Input: part model. Units: mm. Frame: model coordinates. Face numbers are marked on the shaded views. Round coordinates to 2 decimals unless told otherwise and drop trailing zeros. Answer as CSV lines item,"result". Start each with the question number.
1) Line query: L1, parallel to Z at x = -240, y = 2.7. Output: solid intervals per line, ascending.
2) Mould query, pull axis Y, two halves, no side actions, for the marked faces 1 and 2. Classes: +Y half, -Y half, draft (parallel to the pull), parting line (faces both ways), or undercut.
3) First-contact query: P1, Ø6.5, axis at x = 160, z = -100, coming from the -Y side; P2, Ø9, axis at x = 320, z = -100, coming from the -Y side. Flat tips, straight axial feed; report the tip coordinate or a pass-through.
```python
from build123d import *

# Parameters (mm, degrees)
SKETCH1_W                                    = 760
SKETCH1_H                                    = 250
BOSS_EXTRUDE1_DEPTH                          = 3
CSK_FOR_M5_COUNTERSUNK_FLAT_HEAD_SCR_2_COUNT = 2
CSK_FOR_M5_COUNTERSUNK_FLAT_HEAD_SCR_2_PITCH = 80
CSK_FOR_M5_COUNTERSUNK_FLAT_HEAD_SCR_3_COUNT = 2
CSK_FOR_M5_COUNTERSUNK_FLAT_HEAD_SCR_3_PITCH = 160
CSK_FOR_M5_COUNTERSUNK_FLAT_HEAD_SCR_4_COUNT = 2
CSK_FOR_M5_COUNTERSUNK_FLAT_HEAD_SCR_4_PITCH = 240
CSK_FOR_M5_COUNTERSUNK_FLAT_HEAD_SCR_5_COUNT = 2
CSK_FOR_M5_COUNTERSUNK_FLAT_HEAD_SCR_5_PITCH = 320
CSK_FOR_M5_COUNTERSUNK_FLAT_HEAD_SCR_6_COUNT = 2
CSK_FOR_M5_COUNTERSUNK_FLAT_HEAD_SCR_6_PITCH = 80
CSK_FOR_M5_COUNTERSUNK_FLAT_HEAD_SCR_7_COUNT = 2
CSK_FOR_M5_COUNTERSUNK_FLAT_HEAD_SCR_7_PITCH = 160
CSK_FOR_M5_COUNTERSUNK_FLAT_HEAD_SCR_8_COUNT = 2
CSK_FOR_M5_COUNTERSUNK_FLAT_HEAD_SCR_8_PITCH = 240
CSK_FOR_M5_COUNTERSUNK_FLAT_HEAD_SCR_9_COUNT = 2
CSK_FOR_M5_COUNTERSUNK_FLAT_HEAD_SCR_9_PITCH = 320


with BuildPart() as part:
    # Sketch1 → Boss-Extrude1 (new body)
    with BuildSketch(Plane(origin=(0, 0, 0), x_dir=(1, 0, 0), z_dir=(0, 1, 0))):
        Rectangle(SKETCH1_W, SKETCH1_H)
    extrude(amount=BOSS_EXTRUDE1_DEPTH)

    # Sketch3 → CSK for M5 Countersunk Flat Head Screw1 (revolve, cut)
    with BuildSketch(Plane(origin=(0, 0, -100), x_dir=(0, 0, -1), z_dir=(1, 0, 0))):
        Polygon((0, 0), (0, 3), (2.75, 3), (2.75, 2.45), (5.2, 0), align=None)
    csk_for_m5_countersunk_flat_head_screw1 = revolve(axis=Axis((0, -6.35, -100), (0, 1, 0)), mode=Mode.SUBTRACT)

    # CSK for M5 Countersunk Flat Head Scr 2: CSK for M5 Countersunk Flat Head Screw1 ×2
    with Locations(*[(-i * CSK_FOR_M5_COUNTERSUNK_FLAT_HEAD_SCR_2_PITCH, 0, 0) for i in range(1, CSK_FOR_M5_COUNTERSUNK_FLAT_HEAD_SCR_2_COUNT)]):
        add(csk_for_m5_countersunk_flat_head_screw1, mode=Mode.SUBTRACT)

    # CSK for M5 Countersunk Flat Head Scr 3: CSK for M5 Countersunk Flat Head Screw1 ×2
    with Locations(*[(-i * CSK_FOR_M5_COUNTERSUNK_FLAT_HEAD_SCR_3_PITCH, 0, 0) for i in range(1, CSK_FOR_M5_COUNTERSUNK_FLAT_HEAD_SCR_3_COUNT)]):
        add(csk_for_m5_countersunk_flat_head_screw1, mode=Mode.SUBTRACT)

    # CSK for M5 Countersunk Flat Head Scr 4: CSK for M5 Countersunk Flat Head Screw1 ×2
    with Locations(*[(-i * CSK_FOR_M5_COUNTERSUNK_FLAT_HEAD_SCR_4_PITCH, 0, 0) for i in range(1, CSK_FOR_M5_COUNTERSUNK_FLAT_HEAD_SCR_4_COUNT)]):
        add(csk_for_m5_countersunk_flat_head_screw1, mode=Mode.SUBTRACT)

    # CSK for M5 Countersunk Flat Head Scr 5: CSK for M5 Countersunk Flat Head Screw1 ×2
    with Locations(*[(-i * CSK_FOR_M5_COUNTERSUNK_FLAT_HEAD_SCR_5_PITCH, 0, 0) for i in range(1, CSK_FOR_M5_COUNTERSUNK_FLAT_HEAD_SCR_5_COUNT)]):
        add(csk_for_m5_countersunk_flat_head_screw1, mode=Mode.SUBTRACT)

    # CSK for M5 Countersunk Flat Head Scr 6: CSK for M5 Countersunk Flat Head Screw1 ×2
    with Locations(*[(i * CSK_FOR_M5_COUNTERSUNK_FLAT_HEAD_SCR_6_PITCH, 0, 0) for i in range(1, CSK_FOR_M5_COUNTERSUNK_FLAT_HEAD_SCR_6_COUNT)]):
        add(csk_for_m5_countersunk_flat_head_screw1, mode=Mode.SUBTRACT)

    # CSK for M5 Countersunk Flat Head Scr 7: CSK for M5 Countersunk Flat Head Screw1 ×2
    with Locations(*[(i * CSK_FOR_M5_COUNTERSUNK_FLAT_HEAD_SCR_7_PITCH, 0, 0) for i in range(1, CSK_FOR_M5_COUNTERSUNK_FLAT_HEAD_SCR_7_COUNT)]):
        add(csk_for_m5_countersunk_flat_head_screw1, mode=Mode.SUBTRACT)

    # CSK for M5 Countersunk Flat Head Scr 8: CSK for M5 Countersunk Flat Head Screw1 ×2
    with Locations(*[(i * CSK_FOR_M5_COUNTERSUNK_FLAT_HEAD_SCR_8_PITCH, 0, 0) for i in range(1, CSK_FOR_M5_COUNTERSUNK_FLAT_HEAD_SCR_8_COUNT)]):
        add(csk_for_m5_countersunk_flat_head_screw1, mode=Mode.SUBTRACT)

    # CSK for M5 Countersunk Flat Head Scr 9: CSK for M5 Countersunk Flat Head Screw1 ×2
    with Locations(*[(i * CSK_FOR_M5_COUNTERSUNK_FLAT_HEAD_SCR_9_PITCH, 0, 0) for i in range(1, CSK_FOR_M5_COUNTERSUNK_FLAT_HEAD_SCR_9_COUNT)]):
        add(csk_for_m5_countersunk_flat_head_screw1, mode=Mode.SUBTRACT)


solid = part.part
```
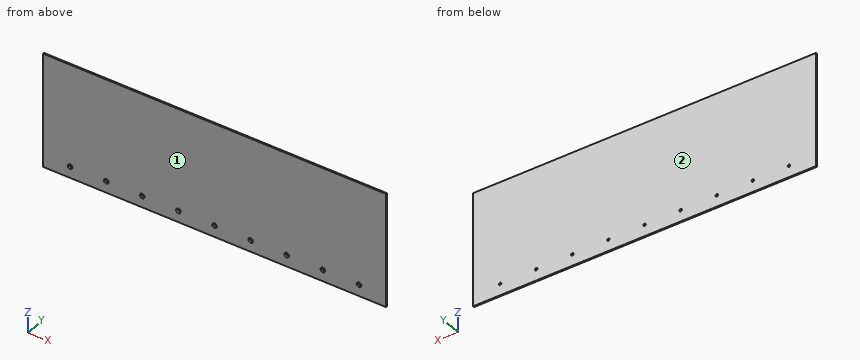
Findings:
1,L1,"z = -125 to -102.75, -97.25 to 125"
2,face 1,"-Y half"
2,face 2,"+Y half"
3,P1,"stops at y = 1.95"
3,P2,"stops at y = 0.7"
